```python
from build123d import *

# Parameters (mm, degrees)
F0_W     = 1400
F0_H     = 480
F1_DEPTH = 20
F3_DEPTH = 1400
F4_W     = 1250
F4_H     = 6
F5_DEPTH = 6
F6_W     = 1240
F6_H     = 20
F7_DEPTH = 20


with BuildPart() as f1:
    # F0 (on Top) → F1 (new body)
    with BuildSketch(Plane.XY):
        Rectangle(F0_W, F0_H)
    extrude(amount=F1_DEPTH)

    # F2 (on face) → F3 (cut)
    with BuildSketch(Plane.YZ.offset(700)):
        Polygon((-240, 20), (-240, 0), (-220, 20), align=None)
    extrude(amount=-F3_DEPTH, mode=Mode.SUBTRACT)

    # F4 (on face) → F5 (cut)
    with BuildSketch(Plane.XY.offset(20)):
        with Locations((0, 219)):
            Rectangle(F4_W, F4_H)
    extrude(amount=-F5_DEPTH, mode=Mode.SUBTRACT)

    # F6 (on face) → F7 (cut)
    with BuildSketch(Plane(origin=(0, 0, 0), x_dir=(1, 0, 0), z_dir=(0, 0, -1))):
        with Locations((0, 230)):
            Rectangle(F6_W, F6_H)
    extrude(amount=-F7_DEPTH, mode=Mode.SUBTRACT)


solid = f1.part
```
Source: CAD feature listing. Evaluate the final solid. Frame: model axes, mm. Coordinates: 2 decimals unless noted, no trailing zeros. Loops run counter-clockwise (first coordinate to the right, second up) from the corner with the lowest first, then second, coordinate; pieces in that order, holes last. Notation, with made-up numbers: (30, 10.25) -> (85, 10.25) arc R23 cw to (85, 21.25) -> close; hole circle Ø4 at (15.25, 29). An arc over 180 degrees is marked (long way). One line per item, written item: value. Start each with the question number.
Q1. Line query: line 1 along Y through (x, z) = (303, 14.5); line 2 along Y through (x, z) = (213, 9); line 3 along Y through (x, z) = (640, 12). Output: solid intervals per line, ascending.
Q2. Section query B-B, the plane x = -352. Return the cut outline in (y, z).
Q3. Contact query for flat-ended pins moving along their axis: P1, Ø3, axis at x = 93, y = 218.5, coming from the +Z side; P2, Ø5, axis at x = 269.5, z = 16, coming from the -Y side. Output: stop coordinate, or through.
Q4. Section query A-A, the plane z = 5.25. Return the cut outline in (x, y).
Results:
1. line 1: -220 to 216, 222 to 240
1. line 2: -220 to 240
1. line 3: -228 to 240
2. outline: (-220, 0) -> (240, 0) -> (240, 20) -> (222, 20) -> (222, 14) -> (216, 14) -> (216, 20) -> (-220, 20) -> close
3. P1: z = 14
3. P2: y = -220
4. outline: (-700, -234.75) -> (-620, -234.75) -> (-620, -220) -> (620, -220) -> (620, -234.75) -> (700, -234.75) -> (700, 240) -> (-700, 240) -> close
